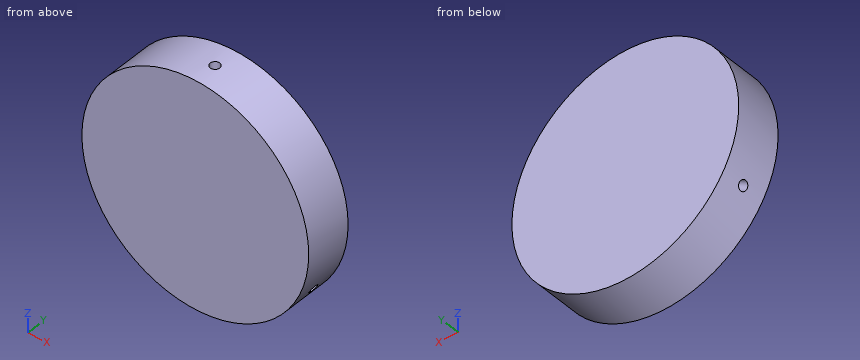
Autodesk Inventor part; units mm, degrees
ref_plane "YZ Plane" through (0, 0, 0) normal (1, 0, 0) x (0, 1, 0)
ref_plane "XZ Plane" through (0, 0, 0) normal (0, 1, 0) x (-1, 0, 0)
sketch "Sketch1" plane through (0, 0, 0) normal (0, 1, 0) x (-1, 0, 0)
  circle A0 centre (0, 0) radius 76.2
  dimension "d0" = 152.4
extrude "Extrusion1" add sketch "Sketch1" along normal blind 31.75
ref_plane "Work Plane1" through (0, 0, 76.2) normal (0, 0, 1) x (1, 0, 0)
sketch "Sketch2" plane through (0, 0, 76.2) normal (0, 0, 1) x (1, 0, 0)
  point P0 (0, 0)
  point P1 (0, 15.875)
  dimension "d4" = 15.875
hole "Hole1" at (0, 15.875, 76.2) direction (0, 0, -1) diameter 6.4008 depth 25.4 tip angle 118
pattern_circular "Circular Pattern1" count 3 over 360 about axis through (0, 31.75, 0) along (0, 1, 0) of "Hole1"
properties part number "Heat-Sink"
The listing builds one solid part. Answer for the finished solid, in the listing's coordinates (mm). Coordinates: 2 decimals unless noted, no trailing zeros. Order: outer loops, then holes, each group sorted by start corner. A loop starts at its lowest first (then second) coordinate and runs counter-clockwise, first axis right, second up.
Q1. Given P1, Ø6, axis at y = 16.5, z = 33.5, coming from the +X side; P2, Ø2, axis at x = -45, y = 22.5, coming from the -Z side; P3, Ø6, axis at y = 28, z = -43.5, coming from the +X side, each flat-ended and moving along its own axis, determine where each tip first touches the part or whether it passes through.
Q2. Consider line 1 (Y direction, x = 0, z = 64); line 2 (X direction, y = 8, z = -20.5); line 3 (Z direction, x = 58.5, y = 13.5). Determine where each line is inside the solid, lowest interval first.
Q3. A cutting plane is placed at C-C, the plane y = 8. Write down the section's boundary in (x, z), and give its area (3 significant figures).
Q4. A cutting plane is placed at A-A, the plane z = 59.5. Write down the section's boundary in (x, y) (3 decimals).
Q5. A cutting plane is placed at B-B, the plane x = 23.5. Write down the section's boundary in (y, z).
Q6. A cutting plane is placed at D-D, the plane z = 35.5. Write down the section's boundary in (x, y).
Answers follow:
1. P1: stops at x = 69.83
1. P2: stops at z = -62.21
1. P3: stops at x = 64.55
2. line 1: y = 0 to 12.67, 19.08 to 31.75
2. line 2: x = -73.39 to 73.39
2. line 3: z = -48.83 to -36.25, -31.3 to 48.83
3. outline: circle Ø152.4 at (0, 0)
3. area: 18,200 mm2
4. outline: (-47.605, 0) - (47.605, 0) - (47.605, 31.75) - (-47.605, 31.75) - close; hole circle Ø6.401 at (0, 15.875)
5. outline: (0, -72.49) - (31.75, -72.49) - (31.75, 72.49) - (0, 72.49) - close
6. outline: (-67.43, 0) - (67.43, 0) - (67.43, 31.75) - (-67.43, 31.75) - close
